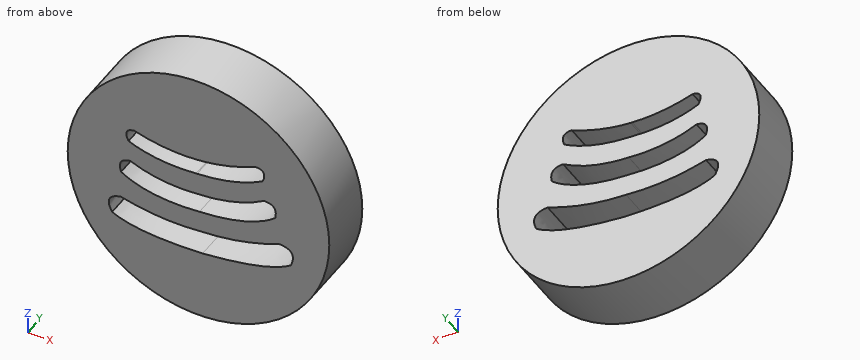
```python
from build123d import *

# Parameters (mm, degrees)
SKETCH1_R           = 4.510832166
BOSS_EXTRUDE1_DEPTH = 2


with BuildPart() as part:
    # Sketch1 → Boss-Extrude1 (new body)
    with BuildSketch(Plane(origin=(0, 0, 0), x_dir=(1, 0, 0), z_dir=(0, 1, 0))):
        with Locations((4.847257792, 4.635414513)):
            Circle(SKETCH1_R)
        with BuildLine():
            Line((4.765839993, 3.704152946), (4.801053978, 3.701743172))
            add(Edge.make_bspline(
                [(4.801053978, 3.701743172), (6.14048774, 3.63517676), (7.067136471, 3.075228485)],
                knots=[0, 0, 0, 1, 1, 1], degree=2))
            add(Edge.make_bspline(
                [(7.067136471, 3.075228485), (7.229894904, 2.616221828), (6.804254242, 2.628959028)],
                knots=[0, 0, 0, 1, 1, 1], degree=2))
            add(Edge.make_bspline(
                [(6.804254242, 2.628959028), (5.8095543, 3.091031812), (4.77441326, 3.163396408)],
                knots=[0, 0, 0, 1, 1, 1], degree=2))
            Line((4.77441326, 3.163396408), (4.718895199, 3.167195635))
            add(Edge.make_bspline(
                [(2.635172404, 2.914258811), (3.683546068, 3.236519406), (4.718895199, 3.167195635)],
                knots=[0, 0, 0, 1, 1, 1], degree=2))
            add(Edge.make_bspline(
                [(2.43553462, 3.392179568), (2.211764545, 2.959623939), (2.635172404, 2.914258811)],
                knots=[0, 0, 0, 1, 1, 1], degree=2))
            add(Edge.make_bspline(
                [(4.765839993, 3.704152946), (3.429824714, 3.820673616), (2.43553462, 3.392179568)],
                knots=[0, 0, 0, 1, 1, 1], degree=2))
        make_face(mode=Mode.SUBTRACT)
        with BuildLine():
            Line((4.833097784, 4.473451505), (4.839222124, 4.473032403))
            add(Edge.make_bspline(
                [(7.101962805, 3.824170948), (6.157905723, 4.415694672), (4.839222124, 4.473032403)],
                knots=[0, 0, 0, 1, 1, 1], degree=2))
            add(Edge.make_bspline(
                [(7.496384151, 4.321712857), (7.596066747, 3.809653625), (7.101962805, 3.824170948)],
                knots=[0, 0, 0, 1, 1, 1], degree=2))
            add(Edge.make_bspline(
                [(4.881790421, 5.14003934), (6.140415114, 5.08430185), (7.038587479, 4.73304729), (7.496384151, 4.321712857)],
                knots=[0, 0, 0, 0, 1, 1, 1, 1], degree=3))
            add(Edge.make_bspline(
                [(4.881790421, 5.14003934), (3.627306072, 5.256279636), (2.689656518, 5.030654558), (2.180092864, 4.6855188)],
                knots=[0, 0, 0, 0, 1, 1, 1, 1], degree=3))
            add(Edge.make_bspline(
                [(2.180092864, 4.6855188), (2.011583443, 4.19181256), (2.503058846, 4.138884439)],
                knots=[0, 0, 0, 1, 1, 1], degree=2))
            add(Edge.make_bspline(
                [(2.503058846, 4.138884439), (3.518896422, 4.5962881), (4.833097784, 4.473451505)],
                knots=[0, 0, 0, 1, 1, 1], degree=2))
        make_face(mode=Mode.SUBTRACT)
        with BuildLine():
            add(Edge.make_bspline(
                [(4.98940547, 6.712616582), (2.708473933, 6.819328215), (1.870039434, 6.362412541)],
                knots=[0, 0, 0, 1, 1, 1], degree=2))
            add(Edge.make_bspline(
                [(1.870039434, 6.362412541), (1.529749193, 5.775598177), (2.172520926, 5.654605851)],
                knots=[0, 0, 0, 1, 1, 1], degree=2))
            add(Edge.make_bspline(
                [(2.172520926, 5.654605851), (3.539396322, 6.021113127), (4.93259631, 5.882465099)],
                knots=[0, 0, 0, 1, 1, 1], degree=2))
            add(Edge.make_bspline(
                [(7.635900953, 5.28073429), (6.331696023, 5.830029687), (4.93259631, 5.882465099)],
                knots=[0, 0, 0, 1, 1, 1], degree=2))
            add(Edge.make_bspline(
                [(8.031984733, 5.940736564), (8.289162951, 5.31303607), (7.635900953, 5.28073429)],
                knots=[0, 0, 0, 1, 1, 1], degree=2))
            add(Edge.make_bspline(
                [(4.98940547, 6.712616582), (7.263610448, 6.507609829), (8.031984733, 5.940736564)],
                knots=[0, 0, 0, 1, 1, 1], degree=2))
        make_face(mode=Mode.SUBTRACT)
    extrude(amount=BOSS_EXTRUDE1_DEPTH)


solid = part.part
```
Design review of the part built by this model. Coordinates are the model's own, in mm. Coordinates: 2 decimals unless noted, no trailing zeros. Order: outer loops, then holes, each group sorted by start corner. A loop starts at its lowest first (then second) coordinate and runs counter-clockwise, first axis right, second up.
1) Clearance check with a flat-ended pin moving along its axis: pin 1 (1 mm diameter, centred on x = 1.5, y = 0.5, fed in from -Z). State where the tip first meets the part, or that it passes through.
2) Take a section at A-A, the plane x = 6. State how many separate pieces and enclosed holes the cut face has, and give its area (3 significant figures).
3) Take a section at D-D, the plane x = 1.25. Give the boundary of the cut face in (y, z).
4) Wall thickness on line 1 along Z through (x, y) = (3.5, 1.6); line 2 along Z through (x, y) = (3, 0.95); line 3 along Z through (x, y) = (2, 0.6): over which ranges is each line inside the solid? List them lowest first.
5) Take a section at C-C, the plane z = -7.75. Give the boundary of the cut face in (x, y), and give its area (3 significant figures).
Returned:
1. pin 1: stops at z = -8.13
2. separate pieces: 4
2. enclosed holes: 0
2. area: 13.2 mm2
3. outline: (0, -7.36) - (2, -7.36) - (2, -1.91) - (0, -1.91) - close
4. line 1: z = -8.94 to -6.71, -5.89 to -5.13, -4.44 to -3.68, -3.11 to -0.33
4. line 2: z = -8.75 to -6.67, -5.83 to -5.03, -4.32 to -3.58, -3.01 to -0.52
4. line 3: z = -8.13 to -6.43, -5.7 to -1.14
5. outline: (1.58, 0) - (8.11, 0) - (8.11, 2) - (1.58, 2) - close
5. area: 13.1 mm2
